```python
from build123d import *

# Parameters (mm, degrees)
F0_W      = 30
F0_H      = 20
F1_DEPTH  = 2
F2_R      = 5
F3_DEPTH  = 25
F4_W      = 5
F4_H      = 4
F5_DEPTH  = 2
F6_W      = 5
F6_H      = 4
F7_DEPTH  = 25
F8_R      = 5
F9_DEPTH  = 25
F11_DEPTH = 20
F13_DEPTH = 2
F15_DEPTH = 2


with BuildPart() as f1:
    # F0 (on Front) → F1 (new body)
    with BuildSketch(Plane.XZ):
        with Locations((15, -10)):
            Rectangle(F0_W, F0_H)
    extrude(amount=F1_DEPTH)

    # F2 (on face) → F3 (cut)
    with BuildSketch(Plane.XZ.offset(2)):
        with Locations((10, -10)):
            Circle(F2_R)
    extrude(amount=-F3_DEPTH, mode=Mode.SUBTRACT)

    # F4 (on face) → F5 (join)
    with BuildSketch(Plane.YZ.offset(30)):
        Polygon((-3, -20), (-2, -20), (-2, 0), (-28, 0), (-28, -20), (-8, -20), (-8, -16), (-3, -16), align=None)
        with Locations((-5.5, -18)):
            Rectangle(F4_W, F4_H)
    extrude(amount=-F5_DEPTH)

    # F6 (on face) → F7 (cut)
    with BuildSketch(Plane.YZ.offset(30)):
        with Locations((-8.5, -18)):
            Rectangle(F6_W, F6_H)
    extrude(amount=-F7_DEPTH, mode=Mode.SUBTRACT)

    # F8 (on face) → F9 (cut)
    with BuildSketch(Plane(origin=(28, 0, 0), x_dir=(0, -1, 0), z_dir=(-1, 0, 0))):
        with Locations((18, -10)):
            Circle(F8_R)
    extrude(amount=-F9_DEPTH, mode=Mode.SUBTRACT)

    # F10 (on face) → F11 (join)
    with BuildSketch(Plane(origin=(0, 0, -20), x_dir=(1, 0, 0), z_dir=(0, 0, -1))):
        with BuildLine():
            ThreePointArc((28, 6), (27.414214, 2.585786), (24, 2))
            Line((24, 2), (24, 0))
            Line((24, 0), (30, 0))
            Line((30, 0), (30, 6))
            Line((30, 6), (28, 6))
        make_face()
    extrude(amount=-F11_DEPTH)

    # F12 (on face) → F13 (join)
    with BuildSketch(Plane(origin=(28, 0, 0), x_dir=(0, -1, 0), z_dir=(-1, 0, 0))):
        Polygon((11, -16), (10.881885, -16), (11, -16.118115), align=None)
    extrude(amount=-F13_DEPTH)

    # F14 (on face) → F15 (join)
    with BuildSketch(Plane(origin=(28, 0, 0), x_dir=(0, -1, 0), z_dir=(-1, 0, 0))):
        Polygon((6.06307, -16), (6, -16), (6, -16.06307), align=None)
    extrude(amount=-F15_DEPTH)


solid = f1.part
```
The listing builds one solid part. Answer for the finished solid, in the listing's coordinates (mm). A direction names the side the tool comes from. Coordinates: 2 decimals unless noted, no trailing zeros. Write each loop counter-clockwise with the first axis right and the second up, starting at its lowest first coordinate (ties: lowest second). Pieces come first, ordered by that corner, then holes. Notation, with made-up numbers: M 38.25,14 L 78.25,14 A18 cw 78.25,49 Z; hole C 48,-26 d10. An arc over 180 degrees is marked long. Use a Markdown table: item, result. Add a question column.
1. Section D-D (z = -10) is taken. Give the vertices of the cut face in (x, y), plus the area to 3 significant figures.
2. Given P1, Ø0.6, axis at x = 29.5, y = -9.5, coming from the -Z side, flat-ended and moving along its own axis, determine where the tip first touches the part or whether it passes through.
3. Which of the six approach directions +Z, -Z, +X, -X, +Y, -Y give full straight-line access (tool end or side, diameter ignored) to faces 4 (the flat face through (29, -6, -18)), 5 (the flat face through (18.5, -1.7, -20)), 6 (the flat face through (16, -2, -10))?
4. Straight lines are drawn through the part: line 1 along Z through (x, y) = (10, -1.45); line 2 along X through (y, z) = (-11, -14); line 3 along Y through (x, z) = (18, -5.5). For each, find the intervals that lie inside material, in ascending order. Write a range as [from, to].
5. Section C-C (x = 10) is taken. Give the vertices of the cut face in (y, z).
6. Section A-A (z = -16.75) is taken. Give the vertices of the cut face in (x, y), plus the area to 3 significant figures.
7. Section B-B (y = -18) is taken. Give the vertices of the cut face in (x, z).
8. For a pull along Y with two mould halves and no side action, classify faces 1 (the flat face through (29, -11, -18)), 2 (the flat face through (30, -11, -10)), 3 (the flat face through (29, -28, -10)) as +Y half, -Y half, draft (parallel to the pull), parting line (faces both ways), or undercut.
Data:
| question | item | result |
|---|---|---|
| 1 | outline | M 0,-2 L 5,-2 L 5,0 L 0,0 Z; M 15,-2 L 26.59,-2 A3 cw 28,-3.41 L 28,-13 L 30,-13 L 30,0 L 15,0 Z; M 28,-28 L 30,-28 L 30,-23 L 28,-23 Z |
| 1 | area | 72.8 mm2 |
| 2 | P1 | stops at z = -16 |
| 3 | face 4 | -Z, +X, -X |
| 3 | face 5 | -Z, +X, -X, +Y, -Y |
| 3 | face 6 | +Z, -Z, -X, -Y |
| 4 | line 1 | z = [-20, -15], [-5, 0] |
| 4 | line 2 | x = [28, 30] |
| 4 | line 3 | y = [-2, 0] |
| 5 | outline | M -2,-20 L 0,-20 L 0,-15 L -2,-15 Z; M -2,-5 L 0,-5 L 0,0 L -2,0 Z |
| 6 | outline | M 0,-2 L 26.59,-2 A3 cw 28,-3.41 L 28,-6 L 30,-6 L 30,0 L 0,0 Z; M 28,-28 L 30,-28 L 30,-11 L 28,-11 Z |
| 6 | area | 103 mm2 |
| 7 | outline | M 28,-20 L 30,-20 L 30,-15 L 28,-15 Z; M 28,-5 L 30,-5 L 30,0 L 28,0 Z |
| 8 | face 1 | undercut |
| 8 | face 2 | draft |
| 8 | face 3 | -Y half |
